The listing builds one solid part. Answer for the finished solid, in the listing's coordinates (mm). Coordinates: 2 decimals unless noted, no trailing zeros. Loops run counter-clockwise (first coordinate to the right, second up) from the corner with the lowest first, then second, coordinate; pieces in that order, holes last. Notation, with made-up numbers: (-8, 30) - (28, 30) arc R22 cw to (28, 52) - close; hole circle Ø6 at (26, 0.25). An arc over 180 degrees is marked (long way). Return JSON: item names as keys, results as strings. Group by question number.
1. Section C-C (y = -23.5) is taken. Write down the section's boundary in (x, z).
2. Find the intervals of material crossed by line 1 along Y through (x, z) = (15.24, 0.85) (3 decimals); line 2 along X through (y, z) = (-15.24, 0.9) (3 decimals); line 3 along Z through (x, y) = (50, -35), in increasing order.
3. Section D-D (y = -15.24) is taken. Write down the section's boundary in (x, z) (3 decimals), and give its area (3 significant figures).
4. Each of these flat-tipped pins is pushed along its axis until it touches: P1, Ø1.9, axis at x = 36.5, z = 14.5, coming from the -Y side; P2, Ø4, axis at y = -35.56, z = 35.56, coming from the -X side. Where does it stop, or does it pass through?
```python
from build123d import *

# Parameters (mm, degrees)
F0_W      = 50.8
F0_H      = 50.8
F1_DEPTH  = 50.8
F2_R      = 5.08
F3_R      = 3.175
F4_DEPTH  = 1.27
F5_R      = 3.175
F6_DEPTH  = 1.27
F7_R      = 3.175
F8_DEPTH  = 1.27
F9_R      = 3.175
F10_DEPTH = 1.27
F11_R     = 3.175
F12_DEPTH = 1.27
F13_R     = 3.175
F14_DEPTH = 1.27


with BuildPart() as f1:
    # F0 (on Top) → F1 (new body)
    with BuildSketch(Plane.XY):
        with Locations((25.4, -25.4)):
            Rectangle(F0_W, F0_H)
    extrude(amount=F1_DEPTH)

    # F2
    f2_edges = [f1.edges().sort_by_distance(p)[0] for p in [
        (50.8, -50.8, 25.4),
        (50.8, -25.4, 50.8),
        (50.8, -25.4, 0),
        (25.4, -50.8, 0),
        (25.4, -50.8, 50.8),
        (0, -50.8, 25.4),
        (50.8, 0, 25.4),
        (0, 0, 25.4),
        (25.4, 0, 50.8),
        (25.4, 0, 0),
        (0, -25.4, 50.8),
        (0, -25.4, 0),
    ]]
    fillet(f2_edges, radius=F2_R)

    # F3 (on face) → F4 (cut)
    with BuildSketch(Plane.XY.offset(50.8)):
        with Locations((25.4, -25.4)):
            Circle(F3_R)
    extrude(amount=-F4_DEPTH, mode=Mode.SUBTRACT)

    # F5 (on face) → F6 (cut)
    with BuildSketch(Plane(origin=(0, 0, 0), x_dir=(1, 0, 0), z_dir=(0, 0, -1))):
        with Locations((15.24, 15.24)):
            Circle(F5_R)
        with Locations((35.56, 15.24)):
            Circle(F5_R)
        with Locations((35.56, 35.56)):
            Circle(F5_R)
        with Locations((15.24, 35.56)):
            Circle(F5_R)
        with Locations((15.24, 25.4)):
            Circle(F5_R)
        with Locations((35.56, 25.4)):
            Circle(F5_R)
    extrude(amount=-F6_DEPTH, mode=Mode.SUBTRACT)

    # F7 (on face) → F8 (cut)
    with BuildSketch(Plane.XZ.offset(50.8)):
        with Locations((25.4, 25.4)):
            Circle(F7_R)
        with BuildLine():
            ThreePointArc((38.735, 35.56), (35.56, 38.735), (32.385, 35.56))
            Line((32.385, 35.56), (38.735, 35.56))
        make_face()
        with BuildLine():
            Line((38.735, 35.56), (32.385, 35.56))
            ThreePointArc((32.385, 35.56), (35.56, 32.385), (38.735, 35.56))
        make_face()
        with Locations((35.56, 15.24)):
            Circle(F7_R)
        with Locations((15.24, 35.56)):
            Circle(F7_R)
        with Locations((15.24, 15.24)):
            Circle(F7_R)
    extrude(amount=-F8_DEPTH, mode=Mode.SUBTRACT)

    # F9 (on face) → F10 (cut)
    with BuildSketch(Plane(origin=(0, 0, 0), x_dir=(-1, 0, 0), z_dir=(0, 1, 0))):
        with Locations((-15.24, 35.56)):
            Circle(F9_R)
        with Locations((-35.56, 15.24)):
            Circle(F9_R)
    extrude(amount=-F10_DEPTH, mode=Mode.SUBTRACT)

    # F11 (on face) → F12 (cut)
    with BuildSketch(Plane(origin=(0, 0, 0), x_dir=(0, -1, 0), z_dir=(-1, 0, 0))):
        with Locations((25.4, 25.4)):
            Circle(F11_R)
        with Locations((35.56, 35.56)):
            Circle(F11_R)
        with Locations((15.24, 15.24)):
            Circle(F11_R)
    extrude(amount=-F12_DEPTH, mode=Mode.SUBTRACT)

    # F13 (on face) → F14 (cut)
    with BuildSketch(Plane.YZ.offset(50.8)):
        with Locations((-15.24, 35.56)):
            Circle(F13_R)
        with Locations((-35.56, 35.56)):
            Circle(F13_R)
        with Locations((-35.56, 15.24)):
            Circle(F13_R)
        with Locations((-15.24, 15.24)):
            Circle(F13_R)
    extrude(amount=-F14_DEPTH, mode=Mode.SUBTRACT)


solid = f1.part
```
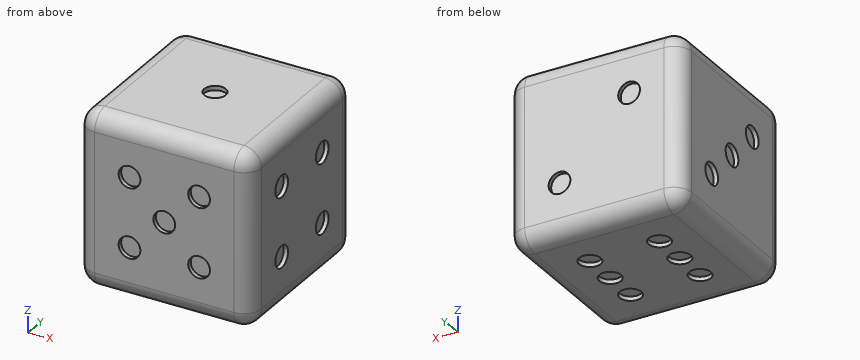
The answers:
{
 "1": {"outline": "(0, 5.08) arc R5.08 ccw to (5.08, 0) - (12.7, 0) - (12.7, 1.27) - (17.78, 1.27) - (17.78, 0) - (33.02, 0) - (33.02, 1.27) - (38.1, 1.27) - (38.1, 0) - (45.72, 0) arc R5.08 ccw to (50.8, 5.08) - (50.8, 45.72) arc R5.08 ccw to (45.72, 50.8) - (27.94, 50.8) - (27.94, 49.53) - (22.86, 49.53) - (22.86, 50.8) - (5.08, 50.8) arc R5.08 ccw to (0, 45.72) - (0, 27.94) - (1.27, 27.94) - (1.27, 22.86) - (0, 22.86) - close"},
 "2": {"line 1": "y = -48.533 to -38.735, -32.385 to -28.575, -22.225 to -18.415, -12.065 to -2.267", "line 2": "x = 2.193 to 12.065, 18.415 to 32.385, 38.735 to 48.607", "line 3": "z = 2.34 to 12.11, 18.37 to 32.43, 38.69 to 48.46"},
 "3": {"outline": "(0, 5.08) arc R5.08 ccw to (5.08, 0) - (12.065, 0) - (12.065, 1.27) - (18.415, 1.27) - (18.415, 0) - (32.385, 0) - (32.385, 1.27) - (38.735, 1.27) - (38.735, 0) - (45.72, 0) arc R5.08 ccw to (50.8, 5.08) - (50.8, 12.065) - (49.53, 12.065) - (49.53, 18.415) - (50.8, 18.415) - (50.8, 32.385) - (49.53, 32.385) - (49.53, 38.735) - (50.8, 38.735) - (50.8, 45.72) arc R5.08 ccw to (45.72, 50.8) - (5.08, 50.8) arc R5.08 ccw to (0, 45.72) - (0, 18.415) - (1.27, 18.415) - (1.27, 12.065) - (0, 12.065) - close", "area": "2,520 mm2"},
 "4": {"P1": "stops at y = -49.53", "P2": "stops at x = 1.27"}
}
